```python
from build123d import *

# Parameters (mm, degrees)
HEADCHAMFER_SIZE = 1.353


with BuildPart() as part:
    # Sketch1 → BaseHead (revolve)
    with BuildSketch(Plane.XY, mode=Mode.PRIVATE) as basehead_sk:
        Polygon((0, 0), (0, 10), (26.25, 10), (30, 9.188), (84.25, 9.188), (88, 10), (130, 10), (130, 0), align=None)
    revolve(basehead_sk.sketch.rotate(Axis((-1.310841664, 0, 0), (1, 0, 0)), 90), axis=Axis((-1.310841664, 0, 0), (1, 0, 0)))

    # HeadChamfer
    headchamfer_edges = [part.edges().sort_by_distance(p)[0] for p in [
        (130, 0, -10),
        (0, 0, -10),
    ]]
    chamfer(headchamfer_edges, length=HEADCHAMFER_SIZE)

    # Sketch2 → BaseBody (revolve)
    with BuildSketch(Plane.XY, mode=Mode.PRIVATE) as basebody_sk:
        Polygon((26.25, 9.188), (30, 10), (84.25, 10), (88, 9.188), align=None)
    revolve(basebody_sk.sketch.rotate(Axis((-1.310841664, 0, 0), (1, 0, 0)), 90), axis=Axis((-1.310841664, 0, 0), (1, 0, 0)))


solid = part.part
```
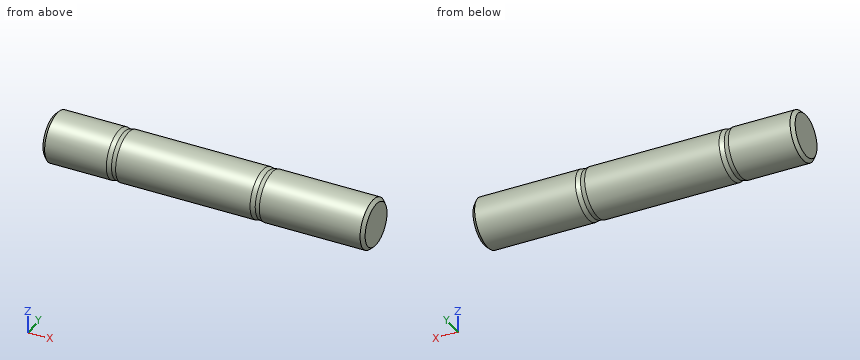
For this review, take the finished solid that the model builds, in its own axes (mm). Coordinates: 2 decimals unless noted, no trailing zeros. Write each loop counter-clockwise with the first axis right and the second up, starting at its lowest first coordinate (ties: lowest second). Pieces come first, ordered by that corner, then holes.
(1) Wall thickness on probe 1 along Z at (x, y) = (15, -5); probe 2 along Z at (x, y) = (27.5, -4.5); probe 3 along Y at (x, z) = (61.5, 0): over which ranges is each line inside the solid? List them lowest first.
(2) Add section A-A on x = 93.5. Give the boundary of the cut face in (y, z), then the cut area to 3 significant figures.
(3) For pin 1 Ø1.5 at (y, z) = (5, -0.5) entering from -X; pin 2 Ø5 at (x, y) = (97.5, 6) entering from -Z; pin 3 Ø6 at (x, y) = (96.5, 5.5) entering from +Z; pin 4 Ø2 at (x, z) = (28.5, -3.5) entering from +Y, all flat-tipped, find the tip position at first contact; note any pin that passes through.
Answer sheet:
1. probe 1: z = -8.66 to 8.66
1. probe 2: z = -8.63 to 8.63
1. probe 3: y = -10 to 10
2. outline: circle Ø20 at (0, 0)
2. area: 314 mm2
3. pin 1: stops at x = 0
3. pin 2: stops at z = -9.37
3. pin 3: stops at z = 9.68
3. pin 4: stops at y = 9.43
